Design review of the part built by this model. Coordinates are the model's own, in mm. A direction names the side the tool comes from. Coordinates: 2 decimals unless noted, no trailing zeros. Loops run counter-clockwise (first coordinate to the right, second up) from the corner with the lowest first, then second, coordinate; pieces in that order, holes last. Notation, with made-up numbers: (65, 33) -> (102, 33) arc R27 cw to (102, 66) -> close; hole circle Ø4 at (52.5, 56). An arc over 180 degrees is marked (long way). Use CSV: the item, a comma, the result in double quotes.
```python
from build123d import *

# Parameters (mm, degrees)
BOSS_EXTRUDE1_DEPTH                    = 25.4
SKETCH21_R                             = 13.97
BOSS_EXTRUDE2_DEPTH                    = 12.7
F_1_2_14_NPSM_TAPPED_HOLE1_D           = 18.9738
F_1_2_14_NPSM_TAPPED_HOLE1_DEPTH       = 25.4
F_1_2_14_NPSM_TAPPED_HOLE1_CSINK_D     = 22.1742
F_1_2_14_NPSM_TAPPED_HOLE1_CSINK_ANGLE = 100
F_1_2_14_NPSM_TAPPED_HOLE1_TIP         = 5.700304607


with BuildPart() as part:
    # Sketch1 → Boss-Extrude1 (new body)
    with BuildSketch(Plane(origin=(0, 0, 0), x_dir=(1, 0, 0), z_dir=(0, 1, 0))):
        with BuildLine():
            Line((-16.51, -37.249073779), (16.51, -37.249073779))
            Line((16.51, -37.249073779), (16.51, -23.558908882))
            Line((16.51, -23.558908882), (22.86, -23.558908882))
            Line((22.86, -23.558908882), (22.86, 0))
            ThreePointArc((22.86, 0), (0, 2.882926221), (-22.86, 0))
            Line((-22.86, 0), (-22.86, -23.558908882))
            Line((-22.86, -23.558908882), (-16.51, -23.558908882))
            Line((-16.51, -23.558908882), (-16.51, -37.249073779))
        make_face()
    extrude(amount=BOSS_EXTRUDE1_DEPTH)

    # Sketch21 → Boss-Extrude2 (add)
    with BuildSketch(Plane.XZ):
        with Locations((0, 22.009073779)):
            Circle(SKETCH21_R)
    extrude(amount=BOSS_EXTRUDE2_DEPTH)

    # 1/2-14 NPSM Tapped Hole1
    with Locations(Plane(origin=(0, 25.4, 0), x_dir=(1, 0, 0), z_dir=(0, 1, 0))):
        with Locations((0, -22.009073779)):
            CounterSinkHole(F_1_2_14_NPSM_TAPPED_HOLE1_D / 2, F_1_2_14_NPSM_TAPPED_HOLE1_CSINK_D / 2, depth=F_1_2_14_NPSM_TAPPED_HOLE1_DEPTH, counter_sink_angle=F_1_2_14_NPSM_TAPPED_HOLE1_CSINK_ANGLE)
            with Locations((0, 0, -(F_1_2_14_NPSM_TAPPED_HOLE1_DEPTH + F_1_2_14_NPSM_TAPPED_HOLE1_TIP / 2))):  # 118° drill point
                Cone(0, F_1_2_14_NPSM_TAPPED_HOLE1_D / 2, F_1_2_14_NPSM_TAPPED_HOLE1_TIP, mode=Mode.SUBTRACT)

    # Sketch26 → Tap Drill for #8-32 Tap1 (revolve, cut)
    with BuildSketch(Plane(origin=(-15.988655959, 12.7, -2.75410008), x_dir=(0, 1, 0), z_dir=(1, 0, 0))):
        Polygon((0, 0), (0, 22.373806461), (1.7272, 21.336), (1.7272, 0), align=None)
    tap_drill_for_8_32_tap1 = revolve(axis=Axis((-15.988655959, 12.7, -9.10410008), (0, 0, 1)), mode=Mode.SUBTRACT)

    # Mirror1: Tap Drill for #8-32 Tap1 across plane
    add(tap_drill_for_8_32_tap1.mirror(Plane(origin=(0, 0, 0), x_dir=(0, 0, 1), z_dir=(1, 0, 0))), mode=Mode.SUBTRACT)


solid = part.part
```
Item 1: Clearance check with flat-ended pins moving along their axes: pin 1 (12 mm diameter, centred on x = -3, y = 17.5, fed in from -Z); pin 2 (3 mm diameter, centred on x = 19.5, y = 15.5, fed in from +Z); pin 3 (6 mm diameter, centred on x = 8.5, y = -5, fed in from +Z); pin 4 (10 mm diameter, centred on y = 15, z = 30.5, fed in from +X). State where each tip first meets the part, or that it passes through.
Checked values:
pin 1,"z = -2.88"
pin 2,"z = 23.56"
pin 3,"z = 34.85"
pin 4,"x = 16.51"
Item 2: Add section B-B (z = 7). Give the boundary of the cut face in (x, y), then the cut area to 3 significant figures.
Checked values:
outline,"(-22.86, 0) -> (22.86, 0) -> (22.86, 25.4) -> (-22.86, 25.4) -> close; hole circle Ø3.45 at (-15.99, 12.7); hole circle Ø3.45 at (15.99, 12.7)"
area,"1,140 mm^2"
Item 3: Add section D-D (y = -9). Give the boundary of the cut face in (x, z), then the cut area to 3 significant figures.
Checked values:
outline,"circle Ø27.94 at (0, 22.01)"
area,"613 mm^2"
Item 4: Add section A-A (y = 23). Give the boundary of the cut face in (x, z) (3 decimals), then the cut area to 3 significant figures.
Checked values:
outline,"(-22.86, 0) arc R92.075 ccw to (22.86, 0) -> (22.86, 23.559) -> (16.51, 23.559) -> (16.51, 37.249) -> (-16.51, 37.249) -> (-16.51, 23.559) -> (-22.86, 23.559) -> close; hole circle Ø18.974 at (0, 22.009)"
area,"1,330 mm^2"
Item 5: Draft analysis for pull direction Y (two halves, no side actions). For faces 1 (the face through (0, 25.4, 8)), 2 (the face through (14.46, 13.5, 8.26)), 3 (the face through (-20, 13, 23.559)), state which applies: pulls with the +Y half, pulls with the -Y half, needs draft (parallel to the pull), parting line crosses it, or undercut.
Checked values:
face 1,"pulls with the +Y half"
face 2,"undercut"
face 3,"needs draft"
Item 6: To check wall thickness, follow line 1 along X through (y, z) = (12.7, 12.25); line 2 along X through (y, z) = (12.7, 14); line 3 along X through (y, z) = (12, 11). State the ranges of each line that lie inside material, in increasing order.
Checked values:
line 1,"-22.86 to -17.72, -14.26 to 14.26, 17.72 to 22.86"
line 2,"-22.86 to -17.72, -14.26 to -5.08, 5.08 to 14.26, 17.72 to 22.86"
line 3,"-22.86 to -17.57, -14.41 to 14.41, 17.57 to 22.86"
Item 7: Add section C-C (x = 13). Give the boundary of the cut face in (y, z), then the cut area to 3 significant figures.
Checked values:
outline,"(-12.7, 16.89) -> (0, 16.89) -> (0, -1.96) -> (25.4, -1.96) -> (25.4, 37.25) -> (0, 37.25) -> (0, 27.12) -> (-12.7, 27.12) -> close"
area,"1,130 mm^2"
Item 8: Machinability: for faces 4 (the face through (-14.46, 13.5, 8.26)), 5 (the face through (-16.51, 13, 30)), 6 (the face through (6.446, -6.261, 9.615)), 7 (the face through (16.51, 13, 30)), which of the approach directions +Z, -Z, +X, -X, +Y, -Y give a long, thin tool a straight path to every point of the face, cutting with its end or side? Answer none if there is none.
Checked values:
face 4,"-Z"
face 5,"+Z, -X, +Y, -Y"
face 6,"-Y"
face 7,"+Z, +X, +Y, -Y"
